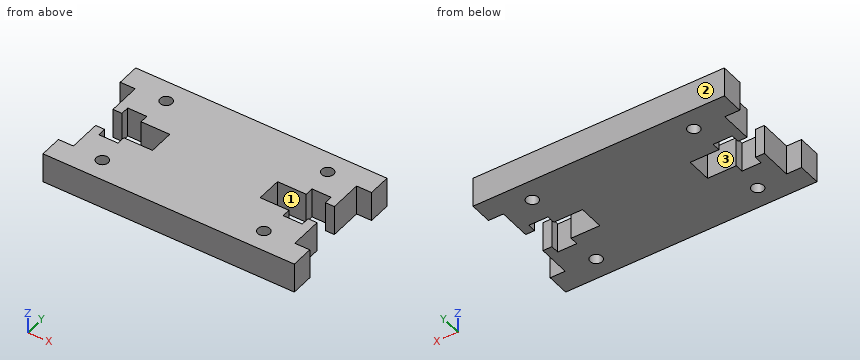
```python
from build123d import *

# Parameters (mm, degrees)
ESQUISSE1_R        = 1
BOSS_EXTRU_1_DEPTH = 5


with BuildPart() as part:
    # Esquisse1 → Boss.-Extru.1 (new body)
    with BuildSketch(Plane.XY):
        Polygon((-7.2, 14.75), (-4, 14.75), (-4, 13.35), (-2.5, 13.35), (-2.5, 18.75), (0, 18.75), (0, 22.5), (-42, 22.5), (-42, 18.75), (-39.5, 18.75), (-39.5, 13.35), (-38, 13.35), (-38, 14.75), (-34.8, 14.75), (-34.8, 13.35), (-30, 13.35), (-30, 9.15), (-34.8, 9.15), (-34.8, 7.75), (-38, 7.75), (-38, 9.15), (-39.5, 9.15), (-39.5, 3.75), (-42, 3.75), (-42, 0), (0, 0), (0, 3.75), (-2.5, 3.75), (-2.5, 9.15), (-4, 9.15), (-4, 7.75), (-7.2, 7.75), (-7.2, 9.15), (-12, 9.15), (-12, 13.35), (-7.2, 13.35), align=None)
        with Locations((-34.5, 3.5)):
            Circle(ESQUISSE1_R, mode=Mode.SUBTRACT)
        with Locations((-7.5, 3.5)):
            Circle(ESQUISSE1_R, mode=Mode.SUBTRACT)
        with Locations((-34.5, 19)):
            Circle(ESQUISSE1_R, mode=Mode.SUBTRACT)
        with Locations((-7.5, 19)):
            Circle(ESQUISSE1_R, mode=Mode.SUBTRACT)
    extrude(amount=BOSS_EXTRU_1_DEPTH)


solid = part.part
```
Geometry: final body of the model. Coordinates: model frame, mm. Face numbers are marked on the shaded views. A direction names the side the tool comes from. Coordinates: 2 decimals unless noted, no trailing zeros. Order: outer loops, then holes, each group sorted by start corner. A loop starts at its lowest first (then second) coordinate and runs counter-clockwise, first axis right, second up. Notation, with made-up numbers: (-6.5, 22.5) -> (43.5, 22.5) arc R10 cw to (43.5, 38.5) -> close; hole circle Ø8 at (71.25, 57.5). An arc over 180 degrees is marked (long way). Write each question's results on one line, items separated by ' | '. Start each with the question number.
1) Material intervals for line 1 along Y through (x, z) = (-7.5, 2); line 2 along Y through (x, z) = (-32.5, 2); line 3 along X through (y, z) = (7.25, 4.1), sorted ascending.
2) Cut plane B-B, the plane x = -34. Output: boundary loops of the cut face in (y, z).
3) Cut plane C-C, the plane z = 1.5. State how many separate pieces and enclosed holes the cut face has, and give its area (3 significant figures).
4) Cut plane D-D, the plane y = 12.25. Output: boundary loops of the cut face in (x, z), and give its area (3 significant figures).
5) First-contact query: pin 1 (1.1 mm diameter, centred on y = 8.5, z = 2, fed in from -X); pin 2 (2 mm diameter, centred on y = 11, z = 1.5, fed in from +X); pin 3 (2.5 mm diameter, centred on y = 17, z = 3.5, fed in from +X). Flat tips, straight axial feed; report the tip coordinate or a pass-through.
6) Set-up query: the marked faces 1, 2 and 3. Return all of +Z, -Z, +X, -X, +Y, -Y with unobstructed straight access to the full face (end or side cutting, diameter ignored); none if empty.
7) Cut plane A-A, the plane x = -39. Output: boundary loops of the cut face in (y, z).
Checks:
1) line 1: 0 to 2.5, 4.5 to 9.15, 13.35 to 18, 20 to 22.5 | line 2: 0 to 9.15, 13.35 to 22.5 | line 3: -39.5 to -2.5
2) outline: (0, 0) -> (2.63, 0) -> (2.63, 5) -> (0, 5) -> close; (4.37, 0) -> (9.15, 0) -> (9.15, 5) -> (4.37, 5) -> close; (13.35, 0) -> (18.13, 0) -> (18.13, 5) -> (13.35, 5) -> close; (19.87, 0) -> (22.5, 0) -> (22.5, 5) -> (19.87, 5) -> close
3) separate pieces: 1 | enclosed holes: 4 | area: 760 mm^2
4) outline: (-30, 0) -> (-12, 0) -> (-12, 5) -> (-30, 5) -> close | area: 90.0 mm^2
5) pin 1: x = -39.5 | pin 2: x = -12 | pin 3: x = -2.5
6) face 1: +Z, -Z, +X | face 2: +Z, -Z, +X, -X, +Y | face 3: +Z, -Z, -X
7) outline: (0, 0) -> (9.15, 0) -> (9.15, 5) -> (0, 5) -> close; (13.35, 0) -> (22.5, 0) -> (22.5, 5) -> (13.35, 5) -> close
